```python
from build123d import *

# Parameters (mm, degrees)
F1_DEPTH = 1
F3_DEPTH = 1
F4_R     = 1.5875
F5_DEPTH = 1


# Not quite as in the source:
# - the program builds the solid bodies; features that only make, move or delete a surface that nothing else refers to are left out


with BuildPart() as f1:
    # F0 (on Top) → F1 (new body)
    with BuildSketch(Plane.XY):
        with BuildLine():
            ThreePointArc((-19.2474145991, 14.2875), (-20.8349145991, 13.862130657), (-21.9970452561, 12.7))
            ThreePointArc((-21.9970452561, 12.7), (-25.4, 0), (-21.9970452561, -12.7))
            ThreePointArc((-21.9970452561, -12.7), (-20.8349145991, -13.862130657), (-19.2474145991, -14.2875))
            Line((-19.2474145991, -14.2875), (19.2474145991, -14.2875))
            ThreePointArc((19.2474145991, -14.2875), (20.8349145991, -13.862130657), (21.9970452561, -12.7))
            ThreePointArc((21.9970452561, -12.7), (25.4, 0), (21.9970452561, 12.7))
            ThreePointArc((21.9970452561, 12.7), (20.8349145991, 13.862130657), (19.2474145991, 14.2875))
            Line((19.2474145991, 14.2875), (-19.2474145991, 14.2875))
        make_face()
    extrude(amount=F1_DEPTH)

    # F2 (on face) → F3 (join)
    with BuildSketch(Plane.XY.offset(1)):
        with BuildLine():
            Line((19.2474145991, 14.2875), (-19.2474145991, 14.2875))
            ThreePointArc((-19.2474145991, 14.2875), (-20.8349145991, 13.862130657), (-21.9970452561, 12.7))
            ThreePointArc((-21.9970452561, 12.7), (-25.4, 0), (-21.9970452561, -12.7))
            ThreePointArc((-21.9970452561, -12.7), (-20.8349145991, -13.862130657), (-19.2474145991, -14.2875))
            Line((-19.2474145991, -14.2875), (19.2474145991, -14.2875))
            ThreePointArc((19.2474145991, -14.2875), (20.8349145991, -13.862130657), (21.9970452561, -12.7))
            ThreePointArc((21.9970452561, -12.7), (25.4, 0), (21.9970452561, 12.7))
            ThreePointArc((21.9970452561, 12.7), (20.8349145991, 13.862130657), (19.2474145991, 14.2875))
        make_face()
        with BuildLine():
            ThreePointArc((-21.4526124879, 11.6252061249), (-20.2856017842, 12.8404540819), (-18.6611352482, 13.2875))
            Line((-18.6611352482, 13.2875), (18.6611352482, 13.2875))
            ThreePointArc((18.6611352482, 13.2875), (20.2856017842, 12.8404540819), (21.4526124879, 11.6252061249))
            ThreePointArc((21.4526124879, 11.6252061249), (24.4, 0), (21.4526124879, -11.6252061249))
            ThreePointArc((21.4526124879, -11.6252061249), (20.2856017842, -12.8404540819), (18.6611352482, -13.2875))
            Line((18.6611352482, -13.2875), (-18.6611352482, -13.2875))
            ThreePointArc((-18.6611352482, -13.2875), (-20.2856017842, -12.8404540819), (-21.4526124879, -11.6252061249))
            ThreePointArc((-21.4526124879, -11.6252061249), (-24.4, 0), (-21.4526124879, 11.6252061249))
        make_face(mode=Mode.SUBTRACT)
    extrude(amount=F3_DEPTH)

    # F4 (on face) → F5 (cut)
    with BuildSketch(Plane.XY.offset(1)):
        with Locations((-21.821282804, 0)):
            Circle(F4_R)
    extrude(amount=-F5_DEPTH, mode=Mode.SUBTRACT)


solid = f1.part
```
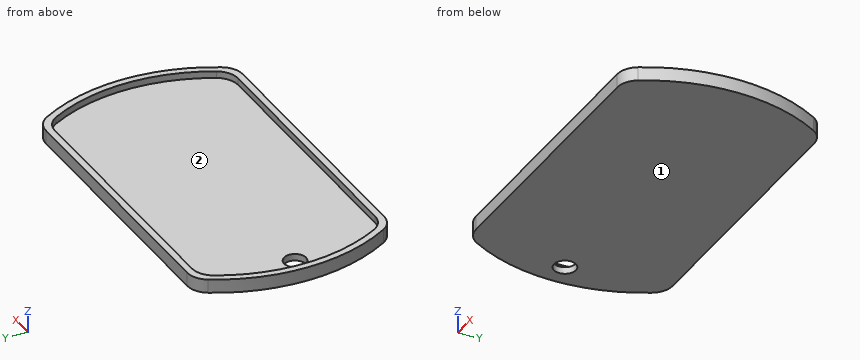
Here's how the part is built. I have some questions about the finished solid (model axes, mm). Face numbers are marked on the shaded views. Give positions to 0.01 mm unless a question says otherwise; leave off trailing zeros. Order: outer loops, then holes, each group sorted by start corner. A loop starts at its lowest first (then second) coordinate and runs counter-clockwise, first axis right, second up. Notation, with made-up numbers: (73.25, 56) -> (102.25, 56) arc R25 ccw to (102.25, 70) -> close; hole circle Ø7 at (3.25, -23). An arc over 180 degrees is marked (long way). Use CSV: the item, a comma, the result in double quotes. Start each with the question number.
Item 1: Suppose I cut it at C-C (x = -17). List the corners of the cut face in (y, z) for me, and give its area (3 significant figures).
Item 2: If I drill on probe 1 along Y at (x, z) = (-10, 1.1); probe 2 along Z at (x, y) = (22, -3.25); probe 3 along X at (y, z) = (1, 0.8), over which ranges is the centre line in solid material (lowest first)? Write a range as [from, to].
Item 3: Thinking about a two-plate mould opening in X: for the marked faces 1 and 2, which applies, pulls with the +X half, pulls with the -X half, needs draft (parallel to the pull), parting line crosses it, or undercut?
Item 4: Suppose I cut it at A-A (y = 0). List the corners of the cut face in (x, z) for me.
Item 5: Suppose I cut it at D-D (x = 20). List the corners of the cut face in (y, z) for me.
Item 6: I'm going to push flat-ended pins straight in: P1, Ø1.9, axis at x = -21.82, y = 0, coming from the -Z side; P2, Ø1, axis at y = 8, z = 1.5, coming from the -X side; P3, Ø1.5, axis at x = -14, y = 5, coming from the +Z side. Where does each tip first touch, or does it pass through?
Answer block:
1,outline,"(-14.29, 0) -> (14.29, 0) -> (14.29, 2) -> (13.29, 2) -> (13.29, 1) -> (-13.29, 1) -> (-13.29, 2) -> (-14.29, 2) -> close"
1,area,"30.6 mm^2"
2,probe 1,"y = [-14.29, -13.29], [13.29, 14.29]"
2,probe 2,"z = [0, 1]"
2,probe 3,"x = [-25.38, -23.05], [-20.59, 25.38]"
3,face 1,"needs draft"
3,face 2,"undercut"
4,outline,"(-25.4, 0) -> (-23.41, 0) -> (-23.41, 1) -> (-24.4, 1) -> (-24.4, 2) -> (-25.4, 2) -> close; (-20.23, 0) -> (25.4, 0) -> (25.4, 2) -> (24.4, 2) -> (24.4, 1) -> (-20.23, 1) -> close"
5,outline,"(-14.2, 0) -> (14.2, 0) -> (14.2, 2) -> (12.99, 2) -> (12.99, 1) -> (-12.99, 1) -> (-12.99, 2) -> (-14.2, 2) -> close"
6,P1,"passes through"
6,P2,"stops at x = -24.27"
6,P3,"stops at z = 1"
